from build123d import *

# Parameters (mm, degrees)
SKETCH_R        = 5
PAD_DEPTH       = 13.25
SKETCH001_R     = 4.1
PAD001_DEPTH    = 7
CHAMFER_SIZE    = 0.25
CHAMFER001_SIZE = 0.25


with BuildPart() as part:
    # Sketch → Pad (new body)
    with BuildSketch(Plane.XY):
        Circle(SKETCH_R)
    extrude(amount=PAD_DEPTH)

    # Sketch001 (on Face3 of Pad) → Pad001 (join)
    with BuildSketch(Plane.XY.offset(13.25)):
        Circle(SKETCH001_R)
    extrude(amount=PAD001_DEPTH)

    # Chamfer
    chamfer_edges = [part.edges().sort_by_distance(p)[0] for p in [
        (-4.1, 0, 20.25),
    ]]
    chamfer(chamfer_edges, length=CHAMFER_SIZE)

    # Chamfer001
    chamfer001_edges = [part.edges().sort_by_distance(p)[0] for p in [
        (-5, 0, 0),
    ]]
    chamfer(chamfer001_edges, length=CHAMFER001_SIZE)


solid = part.part
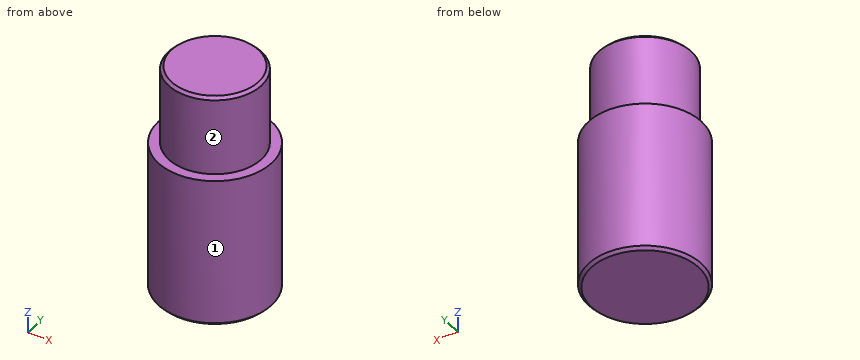
Build history of the part. All positions in model axes, mm. Face numbers are marked on the shaded views. A direction names the side the tool comes from. Coordinates: 2 decimals unless noted, no trailing zeros. Order: outer loops, then holes, each group sorted by start corner. A loop starts at its lowest first (then second) coordinate and runs counter-clockwise, first axis right, second up. Notation, with made-up numbers: (-15, -29) - (27, -29) arc R22 ccw to (27, 1) - close; hole circle Ø4 at (84.25, -38). An arc over 180 degrees is marked (long way). Put each result on its own line as item: value.
1. Drop flat-ended pins along their axis: P1, Ø3, axis at x = 2.5, z = 16, coming from the -Y side; P2, Ø1, axis at x = 2.5, z = 7, coming from the +Y side; P3, Ø1.5, axis at x = 2.5, z = 6, coming from the +Y side. Give the stop position or say it passes through.
Answer sheet:
P1: stops at y = -3.98
P2: stops at y = 4.58
P3: stops at y = 4.68
2. Saw through at C-C (z = 10.5). Write the cut outline in (x, y), and give its area (3 significant figures).
Answer sheet:
outline: circle Ø10 at (0, 0)
area: 78.5 mm^2
3. Saw through at A-A (x = 0). Write the cut outline in (y, z).
Answer sheet:
outline: (-5, 0.25) - (-4.75, 0) - (4.75, 0) - (5, 0.25) - (5, 13.25) - (4.1, 13.25) - (4.1, 20) - (3.85, 20.25) - (-3.85, 20.25) - (-4.1, 20) - (-4.1, 13.25) - (-5, 13.25) - close
4. Tool access for the marked faces 1 and 2: list every direction of +Z, -Z, +X, -X, +Y, -Y with a clear straight run to the whole face (end or side of a thin tool).
Answer sheet:
face 1: +Z, -Z
face 2: +Z
5. Probe line 1 along Z through (x, y) = (4.5, 0.5); line 2 along Y through (x, z) = (-1.25, 3.25); line 3 along Y through (x, z) = (2, 2.25). List the from-to ranges inside material, lowest first. Write a range as [from, to].
Answer sheet:
line 1: z = [0, 13.25]
line 2: y = [-4.84, 4.84]
line 3: y = [-4.58, 4.58]
6. Saw through at D-D (z = 17). Write the cut outline in (x, y), and give its area (3 significant figures).
Answer sheet:
outline: circle Ø8.2 at (0, 0)
area: 52.8 mm^2
